The drawing under review shows one solid part. Ordinate dimensions are in mm from its lowest x, y, z. A direction names the side the tool comes from. Round coordinates to 2 decimals unless told otherwise and drop trailing zeros. Write each loop counter-clockwise with the first axis right and the second up, starting at its lowest first coordinate (ties: lowest second). Pieces come first, ordered by that corner, then holes.
Item 1: Add section B-B (y = 22.5). Give the boundary of the cut face in (x, z), plus the area to 3 significant figures.
Item 2: Machinability: for the marked faces 5 and 6, which of the approach directions +Z, -Z, +X, -X, +Y, -Y give a long, thin tool a straight path to every point of the face, cutting with its end or side? Answer none if there is none.
Item 3: Add section C-C (z = 14.25). Give the boundary of the cut face in (x, y).
Item 4: Draft analysis for pull direction X (two halves, no side actions). For the marked faces 1, 2, 3 and 4, state which applies: +X half, -X half, draft (parallel to the pull), parting line (faces both ways), or undercut.
Item 5: To check wall thickness, follow L1, parallel to Y at x = 60, z = 21.7; L2, parallel to Y at x = 20, z = 24.1; L3, parallel to Z at x = 26, y = 15. State the ranges of each line that lie inside material, in increasing order.
Item 6: Clearance check with flat-ended pins moving along their axes: pin 1 Ø7 at (x, y) = (25.5, 19) entering from +Z; pin 2 Ø2 at (x, z) = (14.5, 4) entering from -Y; pin 3 Ø10 at (y, z) = (35, 20.5) entering from -X. State where each tip first meets the part, or that it passes through.
Item 7: Add section D-D (x = 29.5). Give the boundary of the cut face in (y, z), plus the area to 3 significant figures.
Item 8: Add section A-A (z = 22). Give the boundary of the cut face in (x, y).
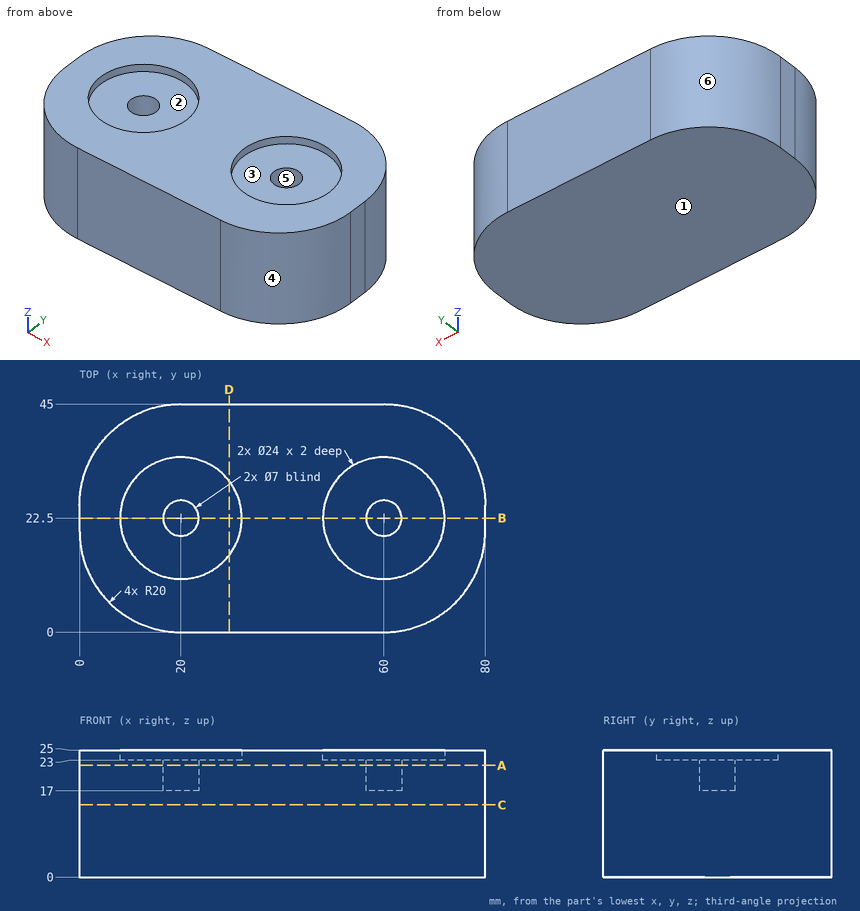
Numbers:
1. outline: (0, 0) - (80, 0) - (80, 25) - (72, 25) - (72, 23) - (63.5, 23) - (63.5, 17) - (56.5, 17) - (56.5, 23) - (48, 23) - (48, 25) - (32, 25) - (32, 23) - (23.5, 23) - (23.5, 17) - (16.5, 17) - (16.5, 23) - (8, 23) - (8, 25) - (0, 25) - close
1. area: 1,820 mm2
2. face 5: +Z
2. face 6: +Z, -Z, -X, +Y
3. outline: (0, 20) arc R20 ccw to (20, 0) - (60, 0) arc R20 ccw to (80, 20) - (80, 25) arc R20 ccw to (60, 45) - (20, 45) arc R20 ccw to (0, 25) - close
4. face 1: draft
4. face 2: undercut
4. face 3: undercut
4. face 4: +X half
5. L1: y = 0 to 19, 26 to 45
5. L2: y = 0 to 10.5, 34.5 to 45
5. L3: z = 0 to 23
6. pin 1: stops at z = 23
6. pin 2: stops at y = 0.51
6. pin 3: stops at x = 0.64
7. outline: (0, 0) - (45, 0) - (45, 25) - (29.83, 25) - (29.83, 23) - (15.17, 23) - (15.17, 25) - (0, 25) - close
7. area: 1,100 mm2
8. outline: (0, 20) arc R20 ccw to (20, 0) - (60, 0) arc R20 ccw to (80, 20) - (80, 25) arc R20 ccw to (60, 45) - (20, 45) arc R20 ccw to (0, 25) - close; hole circle Ø7 at (20, 22.5); hole circle Ø7 at (60, 22.5)
